```python
from build123d import *

# Parameters (mm, degrees)
CYLINDER018_R               = 14.5
CYLINDER018_DEPTH           = 20
CYLINDER114_R               = 2.1
CYLINDER114_DEPTH           = 30
ARRAY001010_X_COUNT         = 2
ARRAY001010_X_PITCH         = 11.3
ARRAY001010_Y_COUNT         = 2
ARRAY001010_Y_PITCH         = 11.3
COMPOUND005_PLACEMENT_ANGLE = 45
CYLINDER012_R               = 4.4
CYLINDER012_DEPTH           = 40
FUSION004_PLACEMENT_ANGLE   = 90
CYLINDER111_R               = 6
CYLINDER111_DEPTH           = 60
BOX011_W                    = 50
BOX011_H                    = 17
BOX011_DEPTH                = 2.2
BOX012_W                    = 50
BOX012_H                    = 12
BOX012_DEPTH                = 60
CYLINDER113_R               = 2.1
CYLINDER113_DEPTH           = 20
ARRAY001019_X_COUNT         = 2
ARRAY001019_X_PITCH         = 13
CYLINDER112_R               = 8.5
CYLINDER112_DEPTH           = 2.2
FUSION013_PLACEMENT_ANGLE   = 90
BOX010_W                    = 7
BOX010_H                    = 56
BOX010_DEPTH                = 36
FILLET005_R                 = 4


with BuildPart() as backlash_nut_disk_hole:
    # Cylinder018 → Cylinder018 (new body)
    with BuildSketch(Plane.XY.offset(-23)):
        Circle(CYLINDER018_R)
    extrude(amount=CYLINDER018_DEPTH)


with BuildPart() as backlash_insert_holes_compound:
    # Cylinder114 → Cylinder114 (new body)
    with BuildSketch(Plane.XY.offset(-20)):
        Circle(CYLINDER114_R)
    extrude(amount=CYLINDER114_DEPTH)

    # Array001010 X: backlash insert holes compound ×2


with BuildPart() as backlash_insert_holes_compound_1:
    add(backlash_insert_holes_compound.part)
    with Locations(*[(i * ARRAY001010_X_PITCH, 0, 0) for i in range(1, ARRAY001010_X_COUNT)]):
        add(backlash_insert_holes_compound.part)

    # Array001010 Y: backlash insert holes compound ×2


with BuildPart() as backlash_insert_holes_compound_2:
    add(backlash_insert_holes_compound_1.part)
    with Locations(*[(0, i * ARRAY001010_Y_PITCH, 0) for i in range(1, ARRAY001010_Y_COUNT)]):
        add(backlash_insert_holes_compound_1.part)


with BuildPart() as backlash_insert_holes_compound_3:
    # Array001010 placement: moved
    add(backlash_insert_holes_compound_2.part.moved(Location((-5.65, -5.65, 0))))


with BuildPart() as backlash_insert_holes_compound_4:
    # Compound005 placement: moved
    add(backlash_insert_holes_compound_3.part.rotate(Axis((0, 0, 0), (0, 0, 1)), COMPOUND005_PLACEMENT_ANGLE))


with BuildPart() as nut_disk_hole_union:
    # Cylinder012 → Cylinder012 (new body)
    with BuildSketch(Plane.XY.offset(-20)):
        Circle(CYLINDER012_R)
    extrude(amount=CYLINDER012_DEPTH)

    # Fusion004: union backlash nut disk hole, backlash insert holes compound
    add(backlash_nut_disk_hole.part)
    add(backlash_insert_holes_compound_4.part)


with BuildPart() as nut_disk_hole_union_1:
    # Fusion004 placement: moved
    add(nut_disk_hole_union.part.moved(Location((6, 17, 16))).rotate(Axis((6, 17, 16), (0, 1, 0)), FUSION004_PLACEMENT_ANGLE))


with BuildPart() as syringe_pusher_body_extract:
    # Cylinder111 → Cylinder111 (new body)
    with BuildSketch(Plane.XY):
        Circle(CYLINDER111_R)
    extrude(amount=CYLINDER111_DEPTH)


with BuildPart() as syringe_pusher_disk_path_extract:
    # Box011 → Box011 (new body)
    with BuildSketch(Plane(origin=(0, -8.5, 60), x_dir=(1, 0, 0), z_dir=(0, 0, 1))):
        with Locations((25, 8.5)):
            Rectangle(BOX011_W, BOX011_H)
    extrude(amount=BOX011_DEPTH)


with BuildPart() as syringe_pusher_body_path_extract:
    # Box012 → Box012 (new body)
    with BuildSketch(Plane(origin=(0, -6, 0), x_dir=(1, 0, 0), z_dir=(0, 0, 1))):
        with Locations((25, 6)):
            Rectangle(BOX012_W, BOX012_H)
    extrude(amount=BOX012_DEPTH)


with BuildPart() as syringe_pusher_insert_hole_extract_array:
    # Cylinder113 → Cylinder113 (new body)
    with BuildSketch(Plane.XY.offset(60)):
        Circle(CYLINDER113_R)
    extrude(amount=CYLINDER113_DEPTH)

    # Array001019 X: syringe pusher insert hole extract array ×2


with BuildPart() as syringe_pusher_insert_hole_extract_array_1:
    add(syringe_pusher_insert_hole_extract_array.part)
    with Locations(*[(i * ARRAY001019_X_PITCH, 0, 0) for i in range(1, ARRAY001019_X_COUNT)]):
        add(syringe_pusher_insert_hole_extract_array.part)


with BuildPart() as middle_block_extract_fusion:
    # Cylinder112 → Cylinder112 (new body)
    with BuildSketch(Plane.XY.offset(60)):
        Circle(CYLINDER112_R)
    extrude(amount=CYLINDER112_DEPTH)

    # Fusion013: union syringe pusher body extract, syringe pusher disk path extract, syringe pusher body path extract, syringe pusher insert hole extract array
    add(syringe_pusher_body_extract.part)
    add(syringe_pusher_disk_path_extract.part)
    add(syringe_pusher_body_path_extract.part)
    add(syringe_pusher_insert_hole_extract_array_1.part)


with BuildPart() as middle_block_extract_fusion_1:
    # Fusion013 placement: moved
    add(middle_block_extract_fusion.part.moved(Location((65.5, 43, 16))).rotate(Axis((65.5, 43, 16), (0, -1, 0)), FUSION013_PLACEMENT_ANGLE))

    # Fusion014: union nut disk hole union
    add(nut_disk_hole_union_1.part)


with BuildPart() as middle_block_cut:
    # Box010 → Box010 (new body)
    with BuildSketch(Plane.XY.offset(-2)):
        with Locations((3.5, 28)):
            Rectangle(BOX010_W, BOX010_H)
    extrude(amount=BOX010_DEPTH)

    # Fillet005
    fillet005_edges = [middle_block_cut.edges().sort_by_distance(p)[0] for p in [
        (3.5, 0, -2),
        (3.5, 0, 34),
        (3.5, 56, -2),
        (3.5, 56, 34),
    ]]
    fillet(fillet005_edges, radius=FILLET005_R)

    # Cut009: cut middle block extract fusion
    add(middle_block_extract_fusion_1.part, mode=Mode.SUBTRACT)


solid = middle_block_cut.part
```
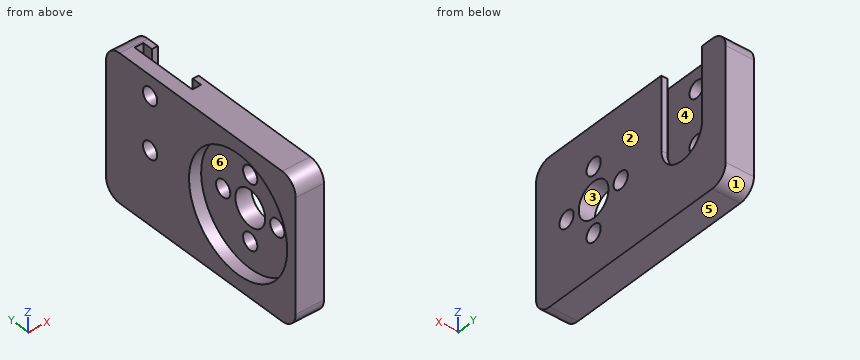
The model under review builds one solid part; all positions refer to its coordinate system, in mm. Face numbers are marked on the shaded views. A direction names the side the tool comes from. Coordinates: 2 decimals unless noted, no trailing zeros. Order: outer loops, then holes, each group sorted by start corner. A loop starts at its lowest first (then second) coordinate and runs counter-clockwise, first axis right, second up. Notation, with made-up numbers: (-35, 35.25) -> (-31, 35.25) arc R20 ccw to (-31, 45.25) -> close; hole circle Ø2 at (74, 2). An arc over 180 degrees is marked (long way). Answer in a Markdown table with one row per item. Add a question column.
Item 1: We need section C-C on z = 9. Write out the cut boundary in (x, y), plus the area to 3 significant figures.
Item 2: We need section D-D on y = 41.5. Write out the cut boundary in (x, z), plus the area to 3 significant figures.
Item 3: Mouldability with a two-part tool opening along Z and no side actions: class the marked faces 1, 2 and 3 as +Z half, -Z half, draft (parallel to the pull), parting line (faces both ways), or undercut.
Item 4: We need section A-A on y = 17. Write out the cut boundary in (x, z), plus the area to 3 significant figures.
Item 5: Machinability: for the marked faces 4, 5 and 6, which of the approach directions +Z, -Z, +X, -X, +Y, -Y give a long, thin tool a straight path to every point of the face, cutting with its end or side? Answer none if there is none.
Item 6: Clearance check with flat-ended pins moving along their axes: pin 1 (5.5 mm diameter, centred on y = 24.99, z = 16, fed in from -X); pin 2 (2.5 mm diameter, centred on y = 43, z = 16, fed in from -X); pin 3 (6.5 mm diameter, centred on y = 43, z = 29, fed in from +X). State where each tip first meets the part, or that it passes through.
Item 7: To check wall thickness, follow probe 1 along Y at (x, z) = (0.75, 16); probe 2 along Z at (x, y) = (4.55, 17); probe 3 along Y at (x, z) = (3.25, 15). State the ranges of each line that lie inside material, in increasing order.
Item 8: We need section B-B on x = 2. Write out the cut boundary in (y, z), plus the area to 3 significant figures.
Final values:
| question | item | result |
|---|---|---|
| 1 | outline | (0, 0) -> (7, 0) -> (7, 15.15) -> (3, 15.15) -> (3, 4.3) -> (0, 4.3) -> close; (0, 29.7) -> (3, 29.7) -> (3, 18.85) -> (7, 18.85) -> (7, 56) -> (0, 56) -> close; hole (3.3, 38.18) -> (5.5, 38.18) -> (5.5, 47.82) -> (3.3, 47.82) -> close |
| 1 | area | 280 mm2 |
| 2 | outline | (0, -2) -> (7, -2) -> (7, 10.19) -> (5.5, 10.19) -> (5.5, 7.63) -> (3.3, 7.63) -> (3.3, 14.53) -> (0, 14.53) -> close; (0, 17.47) -> (3.3, 17.47) -> (3.3, 27.53) -> (0, 27.53) -> close; (0, 30.47) -> (3.3, 30.47) -> (3.3, 34) -> (0, 34) -> close |
| 2 | area | 139 mm2 |
| 3 | face 1 | -Z half |
| 3 | face 2 | draft |
| 3 | face 3 | undercut |
| 4 | outline | (0, -2) -> (7, -2) -> (7, 5.91) -> (3, 5.91) -> (3, 1.5) -> (0, 1.5) -> close; (0, 30.5) -> (3, 30.5) -> (3, 26.09) -> (7, 26.09) -> (7, 34) -> (0, 34) -> close; (3, 10.11) -> (7, 10.11) -> (7, 11.6) -> (3, 11.6) -> close; (3, 20.4) -> (7, 20.4) -> (7, 21.89) -> (3, 21.89) -> close |
| 4 | area | 96.2 mm2 |
| 5 | face 4 | +Z |
| 5 | face 5 | -Z, +X, -X, +Y, -Y |
| 5 | face 6 | -X |
| 6 | pin 1 | stops at x = 3 |
| 6 | pin 2 | passes through |
| 6 | pin 3 | stops at x = 3.3 |
| 7 | probe 1 | y = 0 to 2.5, 31.5 to 40.9, 45.1 to 56 |
| 7 | probe 2 | z = -2 to 5.91, 10.11 to 11.6, 20.4 to 21.89, 26.09 to 34 |
| 7 | probe 3 | y = 0 to 7.16, 10.86 to 12.72, 21.28 to 23.14, 26.84 to 41.15, 44.85 to 56 |
| 8 | outline | (0, 2) arc R4 ccw to (4, -2) -> (52, -2) arc R4 ccw to (56, 2) -> (56, 30) arc R4 ccw to (52, 34) -> (4, 34) arc R4 ccw to (0, 30) -> close; hole circle Ø29 at (17, 16); hole circle Ø4.2 at (43, 16); hole circle Ø4.2 at (43, 29) |
| 8 | area | 1,310 mm2 |
